Geometry: final body of the model. Coordinates: model frame, mm. A direction names the side the tool comes from. Give positions to 0.01 mm unless a question says otherwise; leave off trailing zeros.
Q1. Reachability of faces 4 (the flat face through (-4, -7, 5)), 5 (the flat face through (0, 0, -7.5)) from +Z, -Z, +X, -X, +Y, -Y: full face, straight path, thin tool, end or side. Return the list, or none.
Q2. Mould query, pull axis X, two halves, no side actions, for faces 1 (the flat face through (7, -7, 0)), 2 (the flat face through (1, -7, 5)), 3 (the flat face through (0, 0, 7.5)). Classes: +X half, -X half, draft (parallel to the pull), parting line (faces both ways), or undercut.
Q3. Line query: line 1 (X direction, y = -6.75, z = -1.5); line 2 (Z direction, x = 5.5, y = -6); line 3 (Y direction, x = 4.75, z = 0.5). Output: solid intervals per line, ascending.
Q4. Pin query (flat end, axial travel): pin 1 Ø2.5 at (y, z) = (-7.5, 0) entering from -X; pin 2 Ø2.5 at (y, z) = (-7, 4) entering from +X; pin 3 Ø3 at (x, y) = (-3, -6) entering from -Z. Return the tip coordinate at first contact, or that it passes through.
Q5. Section A-A (y = -6.25). State how many separate pieces and enclosed holes the cut face has, plus the area to 3 significant figures.
from build123d import *

# Parameters (mm, degrees)
SKETCH_1_W                  = 15
SKETCH_1_H                  = 15
EXTRUDE_1_DEPTH             = 4
EXTRUDE_2_DEPTH             = 1
PATTERN_LINEAR_1_COUNT      = 3
PATTERN_LINEAR_1_PITCH      = 3
PATTERN_LINEAR_1_COUNT_DIR2 = 3
PATTERN_LINEAR_1_PITCH_DIR2 = 5
PATTERN_LINEAR_2_COUNT      = 3
PATTERN_LINEAR_2_PITCH      = 3
PATTERN_LINEAR_2_COUNT_DIR2 = 3
PATTERN_LINEAR_2_PITCH_DIR2 = 5


with BuildPart() as part:
    # 스케치1 → 보스-돌출1 (new, symmetric)
    with BuildSketch(Plane(origin=(0, 0, 0), x_dir=(1, 0, 0), z_dir=(0, 1, 0))):
        Rectangle(SKETCH_1_W, SKETCH_1_H)
    extrude(amount=EXTRUDE_1_DEPTH, both=True)

    # 스케치3 → 보스-돌출2 (add, symmetric)
    with BuildSketch(Plane(origin=(0, 0, 0), x_dir=(0, 0, -1), z_dir=(1, 0, 0))):
        with BuildLine():
            Line((2.5, -4), (7.5, -4))
            add(Edge.make_bspline(
                [(6.837946582, -12.278081575), (5.73941202, -8.009656666), (7.5, -4)],
                knots=[0, 0, 0, 1, 1, 1], degree=2))
            add(Edge.make_bspline(
                [(2.5, -4), (2.152812134, -9.664313578), (6.837946582, -12.278081575)],
                knots=[0, 0, 0, 1, 1, 1], degree=2))
        make_face()
    extrude_2 = extrude(amount=EXTRUDE_2_DEPTH, both=True)

    # 선형 패턴1: Extrude 2 3 × 3
    with Locations(*[(-i * PATTERN_LINEAR_1_PITCH, 0, j * PATTERN_LINEAR_1_PITCH_DIR2) for i in range(PATTERN_LINEAR_1_COUNT) for j in range(PATTERN_LINEAR_1_COUNT_DIR2) if (i, j) != (0, 0)]):
        add(extrude_2)

    # 선형 패턴2: Extrude 2 3 × 3
    with Locations(*[(i * PATTERN_LINEAR_2_PITCH, 0, j * PATTERN_LINEAR_2_PITCH_DIR2) for i in range(PATTERN_LINEAR_2_COUNT) for j in range(PATTERN_LINEAR_2_COUNT_DIR2) if (i, j) != (0, 0)]):
        add(extrude_2)


solid = part.part
Computed:
1. face 4: +Z, -Z, -Y
1. face 5: -Z, +X, -X, +Y, -Y
2. face 1: +X half
2. face 2: undercut
2. face 3: draft
3. line 1: x = -7 to -5, -4 to -2, -1 to 1, 2 to 4, 5 to 7
3. line 2: z = -6.8 to -2.54, -1.8 to 2.46, 3.2 to 7.46
3. line 3: y = -4 to 4
4. pin 1: stops at x = -7
4. pin 2: stops at x = 7
4. pin 3: stops at z = -7.29
5. separate pieces: 15
5. enclosed holes: 0
5. area: 125 mm2
